Work out the finished part from the listing and answer in its coordinate system (mm). Round coordinates to 2 decimals unless told otherwise and drop trailing zeros. Order: outer loops, then holes, each group sorted by start corner. A loop starts at its lowest first (then second) coordinate and runs counter-clockwise, first axis right, second up. Notation, with made-up numbers: (36, 1) - (64, 1) arc R18 cw to (64, 36) - close; hole circle Ø1 at (19.25, 27.5). An arc over 180 degrees is marked (long way). Use CSV: the item, a comma, the result in double quotes.
from build123d import *

# Parameters (mm, degrees)
SKETCH1_W          = 0.5
SKETCH1_H          = 8
SKETCH2_W          = 0.2
SKETCH2_H          = 8
CUT_EXTRUDE1_DEPTH = 4


with BuildPart() as part:
    # Sketch1 → Revolve1 (revolve)
    with BuildSketch(Plane.XY, mode=Mode.PRIVATE) as revolve1_sk:
        with Locations((1.75, 4)):
            Rectangle(SKETCH1_W, SKETCH1_H)
    revolve(revolve1_sk.sketch.rotate(Axis((0, 0, 0), (0, 1, 0)), 270), axis=Axis((0, 0, 0), (0, 1, 0)))

    # Sketch2 → Cut-Extrude1 (cut)
    with BuildSketch(Plane(origin=(0, 0, 0), x_dir=(0, 0, -1), z_dir=(1, 0, 0))):
        with Locations((0, 4)):
            Rectangle(SKETCH2_W, SKETCH2_H)
    extrude(amount=CUT_EXTRUDE1_DEPTH, mode=Mode.SUBTRACT)


solid = part.part
(1) Find section B-B (z = -0.9). Determine the outline of the cut face in (x, y).
Findings below:
outline,"(-1.79, 0) - (-1.2, 0) - (-1.2, 8) - (-1.79, 8) - close; (1.2, 0) - (1.79, 0) - (1.79, 8) - (1.2, 8) - close"
(2) Each of these flat-tipped pins is pushed along its axis until it touches: pin 1 (1.5 mm diameter, centred on x = 0.5, y = 7, fed in from +Z); pin 2 (1.8 mm diameter, centred on x = 0, z = 0, fed in from -Y). Where does it stop, or does it pass through?
Findings below:
pin 1,"stops at z = 2"
pin 2,"passes through"
(3) Find section A-A (x = 1.2). Determine the outline of the cut face in (y, z).
Findings below:
outline,"(0, -1.6) - (8, -1.6) - (8, -0.9) - (0, -0.9) - close; (0, 0.9) - (8, 0.9) - (8, 1.6) - (0, 1.6) - close"
(4) Find section D-D (z = 0). Determine the outline of the cut face in (x, y).
Findings below:
outline,"(-2, 0) - (-1.5, 0) - (-1.5, 8) - (-2, 8) - close"
(5) Find section C-C (y = 3.5). Determine the outline of the cut face in (x, z).
Findings below:
outline,"(1.5, -0.1) arc R1.5 cw (long way) to (1.5, 0.1) - (2, 0.1) arc R2 ccw (long way) to (2, -0.1) - close"
(6) Find the intervals of material crossed by L1, parallel to Z at x = 0, y = 2.75; L2, parallel to X at y = 4.25, z = 0; L3, parallel to X at y = 3, z = -1.2, in increasing order. Write a range as from..to.
Findings below:
L1,"z = -2..-1.5, 1.5..2"
L2,"x = -2..-1.5"
L3,"x = -1.6..-0.9, 0.9..1.6"
